Source: CAD feature listing. Evaluate the final solid. Frame: model axes, mm. Face numbers are marked on the shaded views. Round coordinates to 2 decimals unless told otherwise and drop trailing zeros. Loops run counter-clockwise (first coordinate to the right, second up) from the corner with the lowest first, then second, coordinate; pieces in that order, holes last. Notation, with made-up numbers: (-17, -38.75) - (-4, -38.75) arc R30 ccw to (-4, -3.75) - close; hole circle Ø7 at (40, -23.5). An arc over 180 degrees is marked (long way). One line per question, with ' | ' between items.
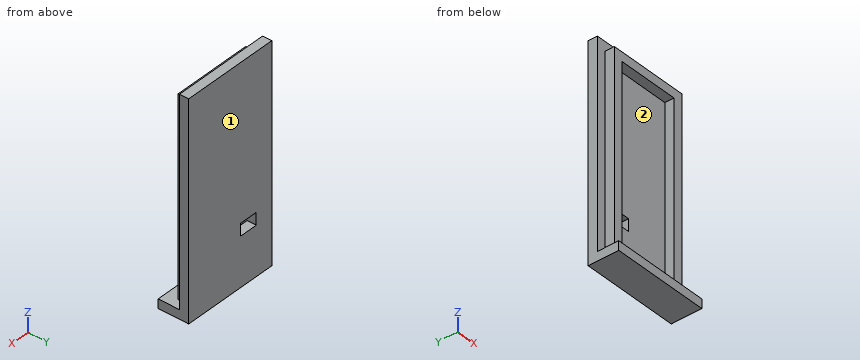
Autodesk Inventor part; units mm, degrees
ref_plane "YZ Plane" through (0, 0, 0) normal (1, 0, 0) x (0, 1, 0)
ref_plane "XZ Plane" through (0, 0, 0) normal (0, 1, 0) x (-1, 0, 0)
ref_plane "XY Plane" through (0, 0, 0) normal (0, 0, 1) x (1, 0, 0)
ref_plane "Płaszczyzna konstrukcyjna1" through (0, 19, 0) normal (0, 1, 0) x (1, 0, 0)
ref_plane "Płaszczyzna konstrukcyjna3" through (0, 19, 0) normal (0, 1, 0) x (1, 0, 0)
ref_plane "Płaszczyzna konstrukcyjna2" through (0, 24, 0) normal (0, 1, 0) x (1, 0, 0)
sketch "Szkic23" plane through (0, 24, 0) normal (0, 1, 0) x (1, 0, 0)
  line L0 (-21.8, -101.1) -> (-21.8, -97.6)
  line L1 (-8.8, -67.6) -> (-8.8, -69.1)
  line L2 (-21.8, -101.1) -> (-8.8, -101.1)
  line L3 (-8.8, -101.1) -> (-8.8, -69.1)
  line L4 (-8.8, -69.1) -> (-21.8, -69.1)
  line L5 (-21.8, -69.1) -> (-21.8, -101.1)
  line L6 (-21.8, -101.1) -> (-20.3, -101.1) construction
  line L7 (-20.3, -101.1) -> (-20.3, -99.6) construction
  line L8 (-20.3, -99.6) -> (-21.8, -99.6) construction
  line L9 (-21.8, -99.6) -> (-21.8, -101.1) construction
  line L10 (-8.8, -69.1) -> (-10.3, -69.1) construction
  line L11 (-21.8, -69.1) -> (-8.8, -69.1) construction
  line L12 (-20.3, -99.6) -> (-10.3, -99.6)
  line L13 (-10.3, -99.6) -> (-10.3, -69.1)
  line L14 (-10.3, -69.1) -> (-20.3, -69.1)
  line L15 (-20.3, -69.1) -> (-20.3, -99.6)
  point P0 (0, 0)
  dimension "d135" = 1.5
  dimension "d136" = 1.5
  dimension "d137" = 1.5
extrude "Wyciągnięcie proste21" add sketch "Szkic23" against normal blind 1.5 contours L0 L5 L4 L15 L12 L13 L3 L2
ref_plane "Płaszczyzna konstrukcyjna5" through (0, 24, 0) normal (0, 1, 0) x (1, 0, 0)
sketch "Szkic24" plane through (0, 24, 0) normal (0, 1, 0) x (1, 0, 0)
  line L0 (-23.3, -69.1) -> (-23.3, -102.6)
  line L1 (-23.3, -69.1) -> (-7.3, -69.1)
  line L2 (-7.3, -69.1) -> (-7.3, -67.6)
  line L3 (-7.3, -67.6) -> (-23.3, -67.6)
  line L4 (-23.3, -67.6) -> (-23.3, -69.1)
  point P0 (0, 0)
  dimension "d140" = 16
  dimension "d141" = 1.5
extrude "Wyciągnięcie proste22" add sketch "Szkic24" against normal blind 3.5
ref_plane "Płaszczyzna konstrukcyjna6" through (0, 24, 0) normal (0, 1, 0) x (1, 0, 0)
sketch "Szkic25" plane through (0, 24, 0) normal (0, 1, 0) x (1, 0, 0)
  line L0 (-7.3, -102.6) -> (-7.3, -69.1)
  line L1 (-23.3, -69.1) -> (-23.3, -67.6)
  line L2 (-7.3, -102.6) -> (-23.3, -102.6)
  line L3 (-23.3, -102.6) -> (-23.3, -67.6)
  line L4 (-23.3, -67.6) -> (-7.3, -67.6)
  line L5 (-7.3, -67.6) -> (-7.3, -102.6)
  point P0 (0, 0)
extrude "Wyciągnięcie proste23" add sketch "Szkic25" along normal blind 1.5
ref_plane "Płaszczyzna konstrukcyjna4" through (0, 20.5, 0) normal (0, 1, 0) x (1, 0, 0)
sketch "Szkic27" plane through (0, 25.5, 0) normal (0, 1, 0) x (1, 0, 0)
  line L0 (-23.3, -67.6) -> (-23.3, -102.6) construction
  line L1 (-23.3, -102.6) -> (-23.3, -77.6) construction
  line L2 (-23.3, -77.6) -> (-23.3, -75.6) construction
  line L3 (-23.3, -77.6) -> (-20.3, -77.6) construction
  line L4 (-23.3, -75.6) -> (-17.3, -75.6) construction
  line L5 (-20.3, -77.6) -> (-17.3, -77.6)
  line L6 (-17.3, -77.6) -> (-17.3, -75.6)
  line L7 (-17.3, -75.6) -> (-20.3, -75.6)
  line L8 (-20.3, -75.6) -> (-20.3, -77.6)
  point P0 (0, 0)
  dimension "d152" = 25
  dimension "d153" = 2
  dimension "d154" = 3
  dimension "d155" = 6
extrude "Wyciągnięcie proste25" cut sketch "Szkic27" against normal blind 10
properties part number "goraczesc1zotworem"
1. Mould query, pull axis X, two halves, no side actions, for the marked faces 1 and 2. Classes: released by +X, released by -X, zero draft, split by the parting line, or undercut.
Worked out:
face 1: zero draft | face 2: undercut
2. Material intervals for probe 1 along X at (y, z) = (24.7, 76.5); probe 2 along Z at (x, y) = (-17.5, 23.05); probe 3 along X at (y, z) = (22.55, 81), sorted ascending.
Worked out:
probe 1: x = -23.3 to -20.3, -17.3 to -7.3 | probe 2: z = 67.6 to 69.1, 99.6 to 101.1 | probe 3: x = -21.8 to -20.3, -10.3 to -8.8
3. Section query A-A, the plane y = 22.85. Return loops of the section in (x, z), plus the area to 3 significant figures.
Worked out:
outline: (-23.3, 67.6) - (-7.3, 67.6) - (-7.3, 69.1) - (-8.8, 69.1) - (-8.8, 101.1) - (-21.8, 101.1) - (-21.8, 69.1) - (-23.3, 69.1) - close; hole (-20.3, 69.1) - (-10.3, 69.1) - (-10.3, 99.6) - (-20.3, 99.6) - close | area: 135 mm2
4. Contact query for flat-ended pins moving along their axis: P1, Ø1, axis at x = -19.5, z = 78, coming from the -Y side; P2, Ø5, axis at x = -12, z = 94, coming from the -Y side; P3, Ø1.2, axis at y = 23, z = 85, coming from the -X side. Output: stop coordinate, or through.
Worked out:
P1: stops at y = 24 | P2: stops at y = 22.5 | P3: stops at x = -21.8
5. Section query B-B, the plane x = -16.5. Return loops of the section in (y, z), plus the area to 3 significant figures.
Worked out:
outline: (20.5, 67.6) - (25.5, 67.6) - (25.5, 102.6) - (24, 102.6) - (24, 101.1) - (22.5, 101.1) - (22.5, 99.6) - (24, 99.6) - (24, 69.1) - (20.5, 69.1) - close | area: 60.0 mm2
6. Section query C-C, the plane z = 81. Return loops of the section in (x, y).
Worked out:
outline: (-23.3, 24) - (-21.8, 24) - (-21.8, 22.5) - (-20.3, 22.5) - (-20.3, 24) - (-10.3, 24) - (-10.3, 22.5) - (-8.8, 22.5) - (-8.8, 24) - (-7.3, 24) - (-7.3, 25.5) - (-23.3, 25.5) - close
